Here's how the part is built. I have some questions about the finished solid (model axes, mm). Round coordinates to 2 decimals unless told otherwise and drop trailing zeros. Loops run counter-clockwise (first coordinate to the right, second up) from the corner with the lowest first, then second, coordinate; pieces in that order, holes last. Notation, with made-up numbers: M 62.5,51 L 88.5,51 A9 ccw 88.5,68 Z; hole C -7.5,-7 d1. An arc over 180 degrees is marked long. Use a Markdown table: item, result.
```python
from build123d import *

# Parameters (mm, degrees)
F0_R     = 13.515014
F1_DEPTH = 2.54
F2_R     = 5.08
F3_DEPTH = 12.192


with BuildPart() as f1:
    # F0 (on Top) → F1 (new body)
    with BuildSketch(Plane.XY):
        with BuildLine():
            ThreePointArc((-42.973429, 36.785428), (-22.173248, 24.273337), (-6.4596, 42.774181))
            ThreePointArc((-6.4596, 42.774181), (-28.242016, 61.275024), (-42.973429, 36.785428))
        make_face()
        with Locations((-25.207632, 42.774181)):
            Circle(F0_R, mode=Mode.SUBTRACT)
        with BuildLine():
            Line((-6.4596, -55.071786), (-6.4596, 42.774181))
            ThreePointArc((-6.4596, 42.774181), (-22.173248, 24.273337), (-42.973429, 36.785428))
            Line((-42.973429, 36.785428), (-11.929202, -55.308118))
            ThreePointArc((-11.929202, -55.308118), (-9.105606, -57.244995), (-6.4596, -55.071786))
        make_face()
    extrude(amount=F1_DEPTH)

    # F2 (on face) → F3 (cut)
    with BuildSketch(Plane.XY.offset(2.54)):
        with Locations((-18.436039, 2.048449)):
            Circle(F2_R)
    extrude(amount=-F3_DEPTH, mode=Mode.SUBTRACT)


solid = f1.part
```
Q1. Imagine slicing it at B-B, the plane x = -20. Please give me the cut outline in (y, z), then the cut area to 3 significant figures.
Return value:
| item | result |
|---|---|
| outline | M -31.37,0 L -2.78,0 L -2.78,2.54 L -31.37,2.54 Z; M 6.88,0 L 30.3,0 L 30.3,2.54 L 6.88,2.54 Z; M 55.25,0 L 60.78,0 L 60.78,2.54 L 55.25,2.54 Z |
| area | 146 mm^2 |
Q2. I need wall thicknesses on line 1 (X direction, y = 43, z = 0.15); line 2 (X direction, y = 39, z = 1.15); line 3 (X direction, y = -45, z = 2.3). Which ranges of each line are inside material? Lowest first, please. Write a range as from..to.
Return value:
| item | result |
|---|---|
| line 1 | x = -43.95..-38.72, -11.69..-6.46 |
| line 2 | x = -43.57..-38.18, -12.23..-6.46 |
| line 3 | x = -15.4..-6.46 |
Q3. Will this pin go through, and if not, where does the flat tip stop? P1, Ø1.5, axis at y = 23, z = 1.5, coming from the -X side.
Return value:
| item | result |
|---|---|
| P1 | stops at x = -38.58 |
Q4. Imagine slicing it at A-A, the plane x = -33. Please give me the cut outline in (y, z).
Return value:
| item | result |
|---|---|
| outline | M 7.2,0 L 31.73,0 L 31.73,2.54 L 7.2,2.54 Z; M 53.82,0 L 59.83,0 L 59.83,2.54 L 53.82,2.54 Z |
Q5. Imagine slicing it at D-D, the plane y = -46. Please give me the cut outline in (x, z), then the cut area to 3 significant figures.
Return value:
| item | result |
|---|---|
| outline | M -15.07,0 L -6.46,0 L -6.46,2.54 L -15.07,2.54 Z |
| area | 21.9 mm^2 |
Q6. We'd pull the mould along X, two halves only. Please class faces 1 (the flat face through (-21, 16, 2.54)), 2 (the cylindrical face through (-9.157, -57.247, 1.252)), 3 (the cylindrical face through (-35.169, 51.908, 1.252)), 4 (the cylindrical face through (-13.6, 3.6, 1.3)): pulls with the +X half, pulls with the -X half, needs draft (parallel to the pull), parting line crosses it, or undercut.
Return value:
| item | result |
|---|---|
| face 1 | needs draft |
| face 2 | parting line crosses it |
| face 3 | undercut |
| face 4 | undercut |
Q7. Imagine slicing it at C-C, the plane z = 1.8. Please give me the cut outline in (x, y), then the cut area to 3 significant figures.
Return value:
| item | result |
|---|---|
| outline | M -42.97,36.79 L -11.93,-55.31 A2.85 ccw -6.46,-55.07 L -6.46,42.77 A18.75 ccw long Z; hole C -25.21,42.77 d27.03; hole C -18.44,2.05 d10.16 |
| area | 2,060 mm^2 |
